Part print with two shaded views. Sizes in mm from the minimum x, y, z corner. A direction names the side the tool comes from. Round coordinates to 2 decimals unless told otherwise and drop trailing zeros. Order: outer loops, then holes, each group sorted by start corner. A loop starts at its lowest first (then second) coordinate and runs counter-clockwise, first axis right, second up. Notation, with made-up numbers: (85, -32) - (93, -32) arc R15 cw to (93, -6) - close; hole circle Ø4 at (9, 53.5). An arc over 180 degrees is marked (long way). Write item = value, one per line.
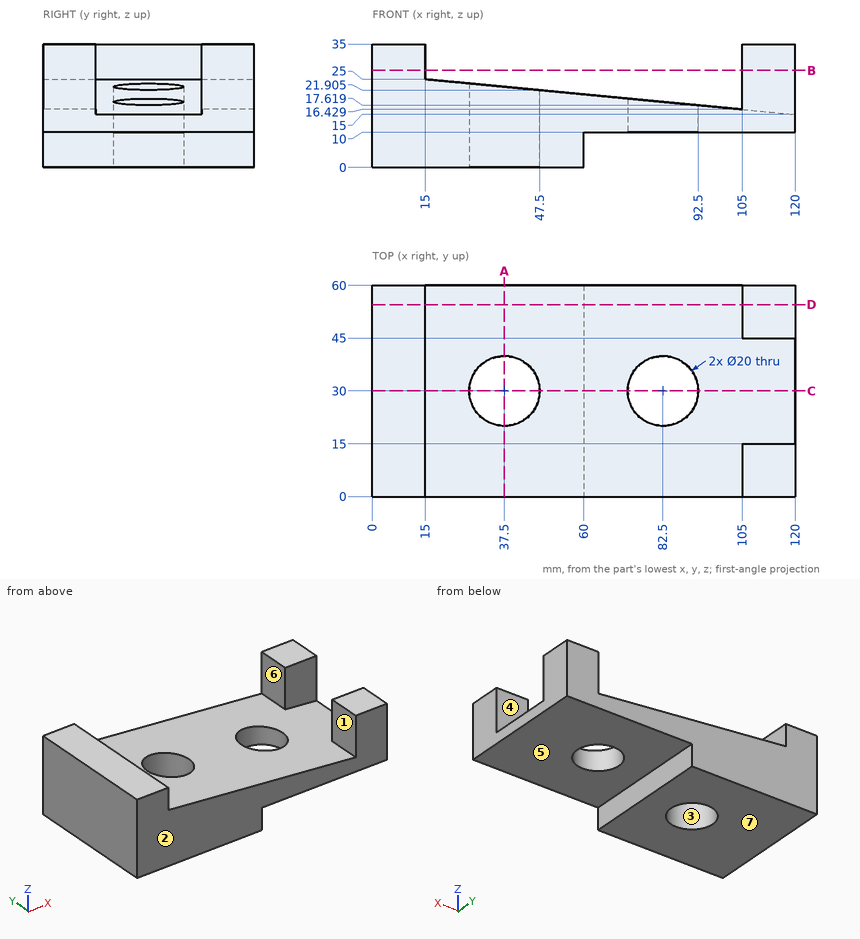
1) 3-axis set-ups, long thin cutter, end or side, ignore diameter. For the marked faces 4, 5, 6 and 7: which of +Z, -Z, +X, -X, +Y, -Y reach the whole face in a straight line?
Conclusion:
face_4 = +Z, +X
face_5 = -Z, +X, +Y, -Y
face_6 = +Z, +Y, -Y
face_7 = -Z, +X, -X, +Y, -Y
2) Mould opens along Y. For the marked faces 1, 2 and 3 say: +Y half, -Y half, draft (parallel to the pull), parting line (faces both ways), or undercut.
Conclusion:
face_1 = draft
face_2 = -Y half
face_3 = undercut
3) Cut at A-A (x = 37.5). Write the cut outline in (y, z), and give its area (3 significant figures).
Conclusion:
outline = (0, 0) - (20, 0) - (20, 22.86) - (0, 22.86) - close; (40, 0) - (60, 0) - (60, 22.86) - (40, 22.86) - close
area = 914 mm^2
4) Cut at D-D (y = 54.5). Write the cut outline in (x, z).
Conclusion:
outline = (0, 0) - (60, 0) - (60, 10) - (120, 10) - (120, 35) - (105, 35) - (105, 16.43) - (15, 25) - (15, 35) - (0, 35) - close
5) Wall check: line 1 along Y through (x, z) = (37.5, 6.75); line 2 along X through (y, z) = (30, 14); line 3 along Y through (x, z) = (113, 26). Give the ranges that are in metal, low to high.
Conclusion:
line_1 = 0 to 20, 40 to 60
line_2 = 0 to 27.5, 47.5 to 72.5, 92.5 to 120
line_3 = 0 to 15, 45 to 60
6) Flat gauge pins, fed straight in: pin 1 Ø3 at (y, z) = (25.5, 6.5) entering from +X; pin 2 Ø2 at (x, y) = (16.5, 25) entering from +Z; pin 3 Ø5 at (y, z) = (22, 30.5) entering from +X. Where does each tip first touch, or does it go through?
Conclusion:
pin_1 = 60
pin_2 = 24.95
pin_3 = 15
7) Cut at B-B (z = 27.5). Write the cut outline in (x, y).
Conclusion:
outline = (0, 0) - (15, 0) - (15, 60) - (0, 60) - close; (105, 0) - (120, 0) - (120, 15) - (105, 15) - close; (105, 45) - (120, 45) - (120, 60) - (105, 60) - close
8) Cut at C-C (y = 30). Write the cut outline in (x, z) (1 decimal).
Conclusion:
outline = (0, 0) - (27.5, 0) - (27.5, 23.8) - (15, 25) - (15, 35) - (0, 35) - close; (47.5, 0) - (60, 0) - (60, 10) - (72.5, 10) - (72.5, 19.5) - (47.5, 21.9) - close; (92.5, 10) - (120, 10) - (120, 15) - (92.5, 17.6) - close
